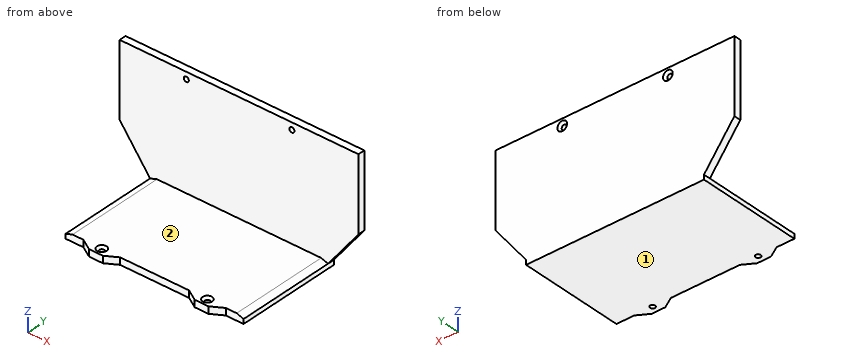
from build123d import *

# Parameters (mm, degrees)
DODANIE_WYCI_GNI_CIE1_DEPTH = 3
DODANIE_WYCI_GNI_CIE2_DEPTH = 43
DODANIE_WYCI_GNI_CIE3_DEPTH = 3
WYTNIJ_WYCI_GNI_CIE2_DEPTH  = 3
SZKIC3_R                    = 1.1
WYTNIJ_WYCI_GNI_CIE3_DEPTH  = 3
SFAZOWANIE1_SIZE            = 1
SFAZOWANIE2_SIZE            = 1


with BuildPart() as part:
    # Szkic1 → Dodanie-wyciągnięcie1 (new body)
    with BuildSketch(Plane(origin=(0, 0, 0), x_dir=(1, 0, 0), z_dir=(0, 1, 0))):
        Polygon((-35.75, -27.18761121), (-38.75, -26.182869049), (-52, -43.745257839), (-52, -75.745257839), (52, -75.745257839), (52, -43.745257839), (38.75, -26.182869049), (35.75, -27.18761121), align=None)
        Polygon((38.75, -24.18761121), (-38.75, -24.18761121), (-38.75, -26.182869049), (-35.75, -27.18761121), (35.75, -27.18761121), (38.75, -26.182869049), align=None)
    extrude(amount=DODANIE_WYCI_GNI_CIE1_DEPTH)

    # Szkic1<3> → Dodanie-wyciągnięcie2 (add)
    with BuildSketch(Plane(origin=(0, 0, 0), x_dir=(1, 0, 0), z_dir=(0, 1, 0))):
        Polygon((38.75, -24.18761121), (-38.75, -24.18761121), (-38.75, -26.182869049), (-35.75, -27.18761121), (35.75, -27.18761121), (38.75, -26.182869049), align=None)
    extrude(amount=-DODANIE_WYCI_GNI_CIE2_DEPTH)

    # Szkic2 → Dodanie-wyciągnięcie3 (add)
    with BuildSketch(Plane.XY.offset(27.18761121)):
        with BuildLine():
            Line((-26, -46), (-20, -46))
            Line((-20, -46), (-20, -43))
            Line((-20, -43), (-21.9, -43))
            ThreePointArc((-21.9, -43), (-23, -44.1), (-24.1, -43))
            Line((-24.1, -43), (-26, -43))
            Line((-26, -43), (-26, -46))
        make_face()
        with BuildLine():
            ThreePointArc((-24.1, -43), (-23, -44.1), (-21.9, -43))
            Line((-21.9, -43), (-24.1, -43))
        make_face()
        with BuildLine():
            Line((-24.1, -43), (-21.9, -43))
            ThreePointArc((-21.9, -43), (-23, -41.9), (-24.1, -43))
        make_face()
        with BuildLine():
            Line((20, -46), (26, -46))
            Line((26, -46), (26, -43))
            Line((26, -43), (24.1, -43))
            ThreePointArc((24.1, -43), (23, -44.1), (21.9, -43))
            Line((21.9, -43), (20, -43))
            Line((20, -43), (20, -46))
        make_face()
        with BuildLine():
            ThreePointArc((21.9, -43), (23, -44.1), (24.1, -43))
            Line((24.1, -43), (21.9, -43))
        make_face()
        with BuildLine():
            Line((21.9, -43), (24.1, -43))
            ThreePointArc((24.1, -43), (23, -41.9), (21.9, -43))
        make_face()
        Polygon((-30.998889877, -43), (-26, -46), (-26, -43), align=None)
        Polygon((-20, -46), (-15.001110123, -43), (-20, -43), align=None)
        Polygon((15.001110123, -43), (20, -46), (20, -43), align=None)
        Polygon((26, -43), (26, -46), (30.998889877, -43), align=None)
    extrude(amount=-DODANIE_WYCI_GNI_CIE3_DEPTH)

    # Szkic2<4> → Wytnij-wyciągnięcie2 (cut)
    with BuildSketch(Plane.XY.offset(27.18761121)):
        with BuildLine():
            ThreePointArc((-24.1, -43), (-23, -44.1), (-21.9, -43))
            Line((-21.9, -43), (-24.1, -43))
        make_face()
        with BuildLine():
            Line((-24.1, -43), (-21.9, -43))
            ThreePointArc((-21.9, -43), (-23, -41.9), (-24.1, -43))
        make_face()
        with BuildLine():
            ThreePointArc((21.9, -43), (23, -44.1), (24.1, -43))
            Line((24.1, -43), (21.9, -43))
        make_face()
        with BuildLine():
            Line((21.9, -43), (24.1, -43))
            ThreePointArc((24.1, -43), (23, -41.9), (21.9, -43))
        make_face()
    extrude(amount=-WYTNIJ_WYCI_GNI_CIE2_DEPTH, mode=Mode.SUBTRACT)

    # Szkic3 → Wytnij-wyciągnięcie3 (cut)
    with BuildSketch(Plane(origin=(0, 3, 0), x_dir=(1, 0, 0), z_dir=(0, 1, 0))):
        with Locations(Location((-23, -72.745257839, 0), (0, 0, 270))):
            Circle(SZKIC3_R)
        with Locations(Location((23, -72.745257839, 0), (0, 0, 270))):
            Circle(SZKIC3_R)
    extrude(amount=-WYTNIJ_WYCI_GNI_CIE3_DEPTH, mode=Mode.SUBTRACT)

    # Sfazowanie1
    sfazowanie1_edges = [part.edges().sort_by_distance(p)[0] for p in [
        (-23, 3, 71.645257839),
    ]]
    chamfer(sfazowanie1_edges, length=SFAZOWANIE1_SIZE)

    # Sfazowanie2
    sfazowanie2_edges = [part.edges().sort_by_distance(p)[0] for p in [
        (23, 3, 71.645257839),
    ]]
    chamfer(sfazowanie2_edges, length=SFAZOWANIE2_SIZE)

    # Sfazowanie3: read off the stored shape, not the designer's step
    # Sfazowanie3 outline → Sfazowanie3 (revolve, cut)
    with BuildSketch(Plane(origin=(23, -43, 0), x_dir=(1, 0, 0), z_dir=(0, -1, 0))):
        Polygon((1.1, 27.18761121), (1.1, 26.18761121), (2.1, 27.18761121), align=None)
    revolve(axis=Axis((23, -43, 0), (0, 0, 1)), mode=Mode.SUBTRACT)

    # Sfazowanie4: read off the stored shape, not the designer's step
    # Sfazowanie4 outline → Sfazowanie4 (revolve, cut)
    with BuildSketch(Plane(origin=(-23, -43, 0), x_dir=(1, 0, 0), z_dir=(0, -1, 0))):
        Polygon((1.1, 27.18761121), (1.1, 26.18761121), (2.1, 27.18761121), align=None)
    revolve(axis=Axis((-23, -43, 0), (0, 0, 1)), mode=Mode.SUBTRACT)


solid = part.part
Part model, mm, in its own coordinate system. Face numbers are marked on the shaded views. A direction names the side the tool comes from. Coordinates: 2 decimals unless noted, no trailing zeros. Order: outer loops, then holes, each group sorted by start corner. A loop starts at its lowest first (then second) coordinate and runs counter-clockwise, first axis right, second up. Notation, with made-up numbers: M 33.5,-16 L 57.5,-16 A19 cw 57.5,11 Z; hole C 20,9 d2. An arc over 180 degrees is marked long. Use a Markdown table: item, result.
(1) Probe L1, parallel to Y at x = -23, z = 25.6; L2, parallel to Z at x = -14, y = -27; L3, parallel to Y at x = -36.5, z = 31. List the from-to ranges inside material, lowest first.
A:
| item | result |
|---|---|
| L1 | y = -46 to -44.1, -41.9 to 3 |
| L2 | z = 24.19 to 27.19 |
| L3 | y = 0 to 3 |
(2) Cut at C-C on x = 9. Write the cut outline in (y, z), then the cut area to 3 significant figures.
A:
| item | result |
|---|---|
| outline | M -43,24.19 L 3,24.19 L 3,75.75 L 0,75.75 L 0,27.19 L -43,27.19 Z |
| area | 284 mm^2 |
(3) Flat gauge pins, fed straight in: pin 1 (2 mm diameter, centred on x = 31, z = 43.5, fed in from -Y); pin 2 (1.8 mm diameter, centred on x = -23, y = -43, fed in from +Z); pin 3 (1.6 mm diameter, centred on y = -12.5, z = 25, fed in from +X); pin 4 (5 mm diameter, centred on x = 22.5, y = -21.5, fed in from +Z). Where does each tip first touch, or does it go through?
A:
| item | result |
|---|---|
| pin 1 | stops at y = 0 |
| pin 2 | passes through |
| pin 3 | stops at x = 38.75 |
| pin 4 | stops at z = 27.19 |
(4) Cut at D-D on z = 36.5. Write the cut outline in (x, y).
A:
| item | result |
|---|---|
| outline | M -46.53,0 L 46.53,0 L 46.53,3 L -46.53,3 Z |
(5) Cut at B-B on z = 66.5. Write the cut outline in (x, y), then the cut area to 3 significant figures.
A:
| item | result |
|---|---|
| outline | M -52,0 L 52,0 L 52,3 L -52,3 Z |
| area | 312 mm^2 |
(6) Tool access for the marked faces 1 and 2: list every direction of +Z, -Z, +X, -X, +Y, -Y with a clear straight run to the whole face (end or side of a thin tool).
A:
| item | result |
|---|---|
| face 1 | -Z, +X, -X, +Y, -Y |
| face 2 | +Z, +X, -X, -Y |
(7) Cut at A-A on x = 23. Write the cut outline in (y, z).
A:
| item | result |
|---|---|
| outline | M -46,24.19 L -44.1,24.19 L -44.1,26.19 L -45.1,27.19 L -46,27.19 Z; M -41.9,24.19 L 3,24.19 L 3,70.65 L 2,71.65 L 0,71.65 L 0,27.19 L -40.9,27.19 L -41.9,26.19 Z; M 0,73.85 L 2,73.85 L 3,74.85 L 3,75.75 L 0,75.75 Z |
